Autodesk Inventor part; units mm, degrees
ref_plane "YZ Plane" through (0, 0, 0) normal (1, 0, 0) x (0, 1, 0)
ref_plane "XZ Plane" through (0, 0, 0) normal (0, 1, 0) x (-1, 0, 0)
ref_plane "XY Plane" through (0, 0, 0) normal (0, 0, 1) x (1, 0, 0)
sketch "Sketch1" plane through (0, 0, 0) normal (0, 0, 1) x (1, 0, 0)
  line L0 (0, 0) -> (620, 0)
  line L1 (110, -188) -> (510, -188)
  line L2 (510, -188) -> (510, -55)
  line L3 (510, -55) -> (620, -55)
  line L4 (620, -55) -> (620, 0)
  line L5 (110, -188) -> (110, -55)
  line L6 (0, -55) -> (0, 0)
  line L7 (0, -55) -> (110, -55)
  point P0 (310, -188)
  point P1 (310, 0)
  dimension "d0" = 620
  dimension "d1" = 188
  dimension "d2" = 400
  dimension "d3" = 133
extrude "Extrusion1" add sketch "Sketch1" along normal blind 10
sketch "Sketch2" plane through (0, 0, 10) normal (0, 0, 1) x (1, 0, 0)
  line L0 (620, 0) -> (0, 0)
  line L1 (510, -188) -> (110, -188)
  line L2 (620, 0) -> (310, 0)
  line L3 (310, 0) -> (310, -188)
  line L4 (310, -188) -> (620, -188)
  line L5 (620, -188) -> (620, 0)
extrude "Extrusion2" cut sketch "Sketch2" against normal through all
sketch "Sketch3" plane through (0, 0, 10) normal (0, 0, 1) x (1, 0, 0)
  circle A0 centre (10, -10) radius 2
  line L0 (310, 0) -> (0, 0)
  line L1 (0, 0) -> (0, -55)
  circle A1 centre (155, -10) radius 2
  circle A2 centre (300, -10) radius 2
  line L2 (310, -188) -> (310, 0)
  line L3 (10, -10) -> (300, -10) construction
  circle A3 centre (120, -178) radius 2
  line L4 (110, -55) -> (110, -188)
  line L5 (110, -188) -> (310, -188)
  circle A4 centre (300, -178) radius 2
  dimension "d8" = 4
  dimension "d9" = 10
  dimension "d10" = 10
  dimension "d11" = 4
  dimension "d12" = 4
  dimension "d13" = 10
  dimension "d14" = 4
  dimension "d15" = 10
  dimension "d16" = 10
  dimension "d17" = 4
  dimension "d18" = 10
  dimension "d19" = 10
extrude "Extrusion3" cut sketch "Sketch3" against normal through all
sketch "Sketch4" plane through (0, 0, 0) normal (0, 0, -1) x (-1, 0, 0)
  line L0 (-310, 0) -> (-310, -188)
  line L1 (-310, -32.5) -> (-328, -32.5)
  line L2 (-328, -32.5) -> (-328, -155.5)
  line L3 (-328, -155.5) -> (-310, -155.5)
  line L4 (-310, -155.5) -> (-310, -32.5)
  circle A0 centre (-320, -46.5) radius 2.5
  circle A1 centre (-320, -141.5) radius 2.5
  line L5 (-320, -46.5) -> (-320, -141.5) construction
  point P0 (0, 0)
  point P1 (-310, -94)
  point P2 (-320, -94)
  dimension "d22" = 18
  dimension "d23" = 123
  dimension "d24" = 5
  dimension "d25" = 5
  dimension "d26" = 10
  dimension "d27" = 95
extrude "Extrusion4" add sketch "Sketch4" against normal blind 5
properties part number "SP001b" material "ABS Plastic"
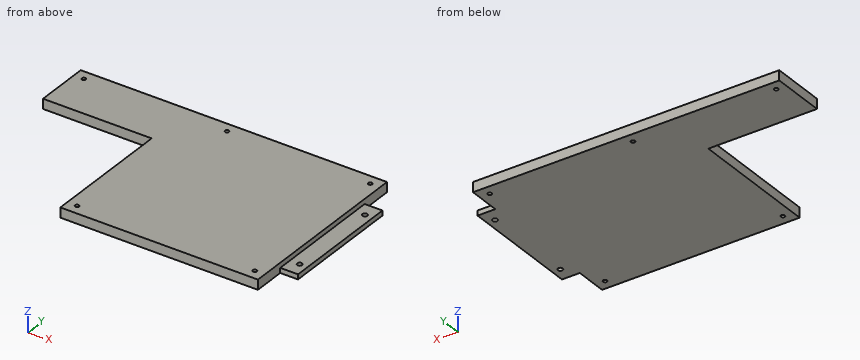
The listing builds one solid part. Answer for the finished solid, in the listing's coordinates (mm). Give positions to 0.01 mm unless a question says otherwise; leave off trailing zeros. Loops run counter-clockwise (first coordinate to the right, second up) from the corner with the lowest first, then second, coordinate; pieces in that order, holes last. Notation, with made-up numbers: (-4.5, 48) - (25.5, 48) arc R31 cw to (25.5, 82) - close; hole circle Ø9 at (-29, 10.25). An arc over 180 degrees is marked (long way). Answer as CSV lines item,"result". Start each with the question number.
Item 1: Each of these flat-tipped pins is pushed along its axis until it touches: pin 1 (2.5 mm diameter, centred on x = 315.5, z = 3.5, fed in from +Y); pin 2 (20 mm diameter, centred on x = 315, y = -97, fed in from +Z); pin 3 (2.5 mm diameter, centred on x = 319.5, z = 2, fed in from -Y); pin 4 (8 mm diameter, centred on x = 320, y = -141.5, fed in from +Z). Where does it stop, or does it pass through?
Item 2: A cutting plane is placed at A-A on z = 1.5. Determine the outline of the cut face in (x, y), then the cut area to 3 significant figures.
Item 3: A cutting plane is placed at B-B on y = -64. Determine the outline of the cut face in (x, z).
Item 4: A cutting plane is placed at D-D on y = -171.5. Determine the outline of the cut face in (x, z).
Item 5: A cutting plane is placed at C-C on x = 29.5. Determine the outline of the cut face in (y, z), then the cut area to 3 significant figures.
Item 6: Find the intervals of material crossed by line 1 (X direction, y = -178, z = 5.75); line 2 (Y direction, x = 320, z = 1.65); line 3 (Y direction, x = 120, z = 4.5), in increasing order. Write a range as from..to.
Found:
1,pin 1,"stops at y = -32.5"
1,pin 2,"stops at z = 10"
1,pin 3,"stops at y = -155.5"
1,pin 4,"stops at z = 5"
2,outline,"(0, -55) - (110, -55) - (110, -188) - (310, -188) - (310, -155.5) - (328, -155.5) - (328, -32.5) - (310, -32.5) - (310, 0) - (0, 0) - close; hole circle Ø4 at (10, -10); hole circle Ø4 at (120, -178); hole circle Ø4 at (155, -10); hole circle Ø4 at (300, -178); hole circle Ø4 at (300, -10); hole circle Ø5 at (320, -141.5); hole circle Ø5 at (320, -46.5)"
2,area,"45,800 mm^2"
3,outline,"(110, 0) - (328, 0) - (328, 5) - (310, 5) - (310, 10) - (110, 10) - close"
4,outline,"(110, 0) - (310, 0) - (310, 10) - (110, 10) - close"
5,outline,"(-55, 0) - (0, 0) - (0, 10) - (-55, 10) - close"
5,area,"550 mm^2"
6,line 1,"x = 110..118, 122..298, 302..310"
6,line 2,"y = -155.5..-144, -139..-49, -44..-32.5"
6,line 3,"y = -188..-180, -176..0"
